```python
from build123d import *

# Parameters (mm, degrees)
BOSS_EXTRUDE1_DEPTH = 3.2
SKETCH2_R           = 15.135
BOSS_EXTRUDE2_DEPTH = 12.2
SKETCH3_R           = 13.5
CUT_EXTRUDE1_DEPTH  = 12.8
SWEEP1_PROFILE_R    = 4
SKETCH29_R          = 4.1
BOSS_EXTRUDE4_DEPTH = 5.7
SKETCH33_W          = 7.16
SKETCH33_H          = 1
BOSS_EXTRUDE5_DEPTH = 18
SKETCH34_R          = 1.5
CUT_EXTRUDE2_DEPTH  = 22.7


with BuildPart() as part:
    # Sketch1 → Boss-Extrude1 (new body)
    with BuildSketch(Plane.XY):
        Polygon((10.796450034, -18.7), (21.592900068, 0), (10.796450034, 18.7), (-10.796450034, 18.7), (-21.592900068, 0), (-10.796450034, -18.7), align=None)
    extrude(amount=BOSS_EXTRUDE1_DEPTH)

    # Sketch2 → Boss-Extrude2 (add)
    with BuildSketch(Plane.XY.offset(3.2)):
        Circle(SKETCH2_R)
    extrude(amount=BOSS_EXTRUDE2_DEPTH)

    # Sketch3 → Cut-Extrude1 (cut)
    with BuildSketch(Plane(origin=(0, 0, 0), x_dir=(-1, 0, 0), z_dir=(0, 0, -1))):
        Circle(SKETCH3_R)
    extrude(amount=-CUT_EXTRUDE1_DEPTH, mode=Mode.SUBTRACT)

    # Sweep1: sweep along a path in Sketch4
    with BuildLine(Plane(origin=(0, 0, 0), x_dir=(1, 0, 0), z_dir=(0, 1, 0))) as sweep1_path:
        Line((-6.135, 0), (-6.135, -115.4))
        ThreePointArc((-6.135, -115.4), (-0.135, -121.4), (5.865, -115.4))
        Line((5.865, -115.4), (5.865, 0))
    # Sweep1 profile (on start of the path) → Sweep1 (sweep)
    with BuildSketch(Plane(origin=(-6.135, 0, 0), x_dir=(1, 0, 0), z_dir=(0, 0, 1))):
        Circle(SWEEP1_PROFILE_R)
    sweep(path=sweep1_path.line)

    # Sketch29 → Boss-Extrude4 (add)
    with BuildSketch(Plane(origin=(0, 0, 0), x_dir=(-1, 0, 0), z_dir=(0, 0, -1))):
        with Locations((-5.865, 0)):
            Circle(SKETCH29_R)
        with Locations((6.135, 0)):
            Circle(SKETCH29_R)
    extrude(amount=BOSS_EXTRUDE4_DEPTH)

    # Sketch33 → Boss-Extrude5 (add)
    with BuildSketch(Plane(origin=(0, 0, -5.7), x_dir=(-1, 0, 0), z_dir=(0, 0, -1))):
        with Locations((-5.88, 2.5)):
            Rectangle(SKETCH33_W, SKETCH33_H)
        with Locations((5.88, 2.5)):
            Rectangle(SKETCH33_W, SKETCH33_H)
    extrude(amount=BOSS_EXTRUDE5_DEPTH)

    # Sketch34 → Cut-Extrude2 (cut, through all)
    with BuildSketch(Plane(origin=(0, 3, 0), x_dir=(1, 0, 0), z_dir=(0, 1, 0))):
        with BuildLine():
            ThreePointArc((-9.46, 20.12), (-8.411442277, 22.651442277), (-5.88, 23.7))
            Line((-5.88, 23.7), (-9.46, 23.7))
            Line((-9.46, 23.7), (-9.46, 20.12))
        make_face()
        with BuildLine():
            ThreePointArc((-5.88, 23.7), (-3.348557723, 22.651442277), (-2.3, 20.12))
            Line((-2.3, 20.12), (-2.3, 23.7))
            Line((-2.3, 23.7), (-5.88, 23.7))
        make_face()
        with BuildLine():
            ThreePointArc((2.3, 20.12), (3.348557723, 22.651442277), (5.88, 23.7))
            Line((5.88, 23.7), (2.3, 23.7))
            Line((2.3, 23.7), (2.3, 20.12))
        make_face()
        with BuildLine():
            ThreePointArc((5.88, 23.7), (8.411442277, 22.651442277), (9.46, 20.12))
            Line((9.46, 20.12), (9.46, 23.7))
            Line((9.46, 23.7), (5.88, 23.7))
        make_face()
        with Locations((-5.88, 20.12)):
            Circle(SKETCH34_R)
        with Locations((5.88, 20.12)):
            Circle(SKETCH34_R)
    extrude(amount=-CUT_EXTRUDE2_DEPTH, mode=Mode.SUBTRACT)


solid = part.part
```
The listing builds one solid part. Answer for the finished solid, in the listing's coordinates (mm). A direction names the side the tool comes from. Coordinates: 2 decimals unless noted, no trailing zeros. Write each loop counter-clockwise with the first axis right and the second up, starting at its lowest first coordinate (ties: lowest second). Pieces come first, ordered by that corner, then holes. Notation, with made-up numbers: (41.5, 42.5) - (96.5, 42.5) arc R8 ccw to (96.5, 51.5) - close; hole circle Ø11 at (77, 14.25). An arc over 180 degrees is marked (long way). Return JSON: item names as keys, results as strings. Group by question number.
1. Which of the six approach directions +Z, -Z, +X, -X, +Y, -Y give full straight-line access (tool end or side, diameter ignored) to faces 5 (the flat face through (-6, 3, -15)), 6 (the cylindrical face through (9.04, -2.43, 6.31)), 7 (the flat face through (-6, 2, -15)), 8 (the cylindrical face through (2.93, -13.18, 6.31)), 9 (the flat face through (-16.12, 9.48, 1.58))?
2. A cutting plane is placed at A-A, the plane z = 68. Determine the outline of the cut face in (x, y) (3 decimals).
3. A cutting plane is placed at B-B, the plane y = 6. Determine the outline of the cut face in (x, z).
4. Straight lines are drawn through the part: L1, parallel to Y at x = 0, z = 3.75 (3 decimals); L2, parallel to Y at x = -3, z = -12; L3, parallel to Z at x = -5.88, y = 2.65. For each, find the intervals that lie inside material, in ascending order.
5. Determine the mould class of faces 1 (the cylindrical face through (9.04, -2.43, 64.7)), 2 (the cylindrical face through (-3.281, -14.775, 9.215)), 3 (the cylindrical face through (-4.29, -3.55, 6.49)), 4 (the flat face through (14, 0, 0)) for opening direction Z: released by +Z, released by -Z, zero draft, split by the parting line, or undercut.
6. Given pin 1 (1 mm diameter, centred on y = 1, z = 19, fed in from +X); pin 2 (10 mm diameter, centred on x = -10, y = 8.5, fed in from -Z); pin 3 (12 mm diameter, centred on x = -12.5, y = 2.5, fed in from -Z), each flat-ended and moving along its own axis, determine where each tip first touches the part or whether it passes through.
Ans:
{
 "1": {"face 5": "-Z, +X, -X, +Y", "face 6": "none", "face 7": "-Z, +X, -X, -Y", "face 8": "-Z", "face 9": "+Z, -Z, -X, +Y"},
 "2": {"outline": "circle Ø8 at (-6.135, 0); circle Ø8 at (5.865, 0)"},
 "3": {"outline": "(-18.13, 0) - (-12.09, 0) - (-12.09, 12.8) - (12.09, 12.8) - (12.09, 0) - (18.13, 0) - (18.13, 3.2) - (13.89, 3.2) - (13.89, 15.4) - (-13.89, 15.4) - (-13.89, 3.2) - (-18.13, 3.2) - close"},
 "4": {"L1": "-15.135 to -13.5, 13.5 to 15.135", "L2": "2 to 3", "L3": "-23.7 to -21.62, -18.62 to 122.32"},
 "5": {"face 1": "undercut", "face 2": "zero draft", "face 3": "undercut", "face 4": "released by -Z"},
 "6": {"pin 1": "x = 9.83", "pin 2": "z = 0", "pin 3": "z = -23.65"}
}
